The model under review builds one solid part; all positions refer to its coordinate system, in mm. Face numbers are marked on the shaded views. A direction names the side the tool comes from. Give positions to 0.01 mm unless a question says otherwise; leave off trailing zeros. Write each loop counter-clockwise with the first axis right and the second up, starting at its lowest first coordinate (ties: lowest second). Pieces come first, ordered by that corner, then holes. Notation, with made-up numbers: (46, -5) - (72, -5) arc R9 cw to (72, 10) - close; hole circle Ø4 at (-28, 85). An arc over 180 degrees is marked (long way). Write item = value, one per line.
```python
from build123d import *

# Parameters (mm, degrees)
SKETCH002_W  = 48.5
SKETCH002_H  = 45
PAD_DEPTH    = 10
SKETCH003_W  = 42.5
SKETCH003_H  = 24.5
PAD002_DEPTH = 3
SKETCH004_W  = 17.5
SKETCH004_H  = 18
PAD003_DEPTH = 12
FILLET_R     = 1
FILLET001_R  = 8.5


with BuildPart() as part:
    # Sketch002 → Pad (new body)
    with BuildSketch(Plane.XZ):
        Rectangle(SKETCH002_W, SKETCH002_H)
    extrude(amount=PAD_DEPTH)

    # Sketch003 (on Face6 of Pad) → Pad002 (join)
    with BuildSketch(Plane.XZ.offset(10)):
        with Locations((0, 8.25)):
            Rectangle(SKETCH003_W, SKETCH003_H)
    extrude(amount=PAD002_DEPTH)

    # Sketch004 (on Face4 of Pad002) → Pad003 (join)
    with BuildSketch(Plane(origin=(0, 0, 0), x_dir=(1, 0, 0), z_dir=(0, 1, 0))):
        with Locations((0, 12)):
            Rectangle(SKETCH004_W, SKETCH004_H)
    extrude(amount=PAD003_DEPTH)

    # Fillet
    fillet_edges = [part.edges().sort_by_distance(p)[0] for p in [
        (24.25, -5, 22.5),
        (24.25, -5, -22.5),
        (-24.25, -5, 22.5),
        (-24.25, -5, -22.5),
    ]]
    fillet(fillet_edges, radius=FILLET_R)

    # Fillet001
    fillet001_edges = [part.edges().sort_by_distance(p)[0] for p in [
        (8.75, 6, -3),
        (-8.75, 6, -3),
    ]]
    fillet(fillet001_edges, radius=FILLET001_R)


with BuildPart() as part_1:
    # Body placement: moved
    add(part.part.moved(Location((0, 10, 0))))


solid = part_1.part
```
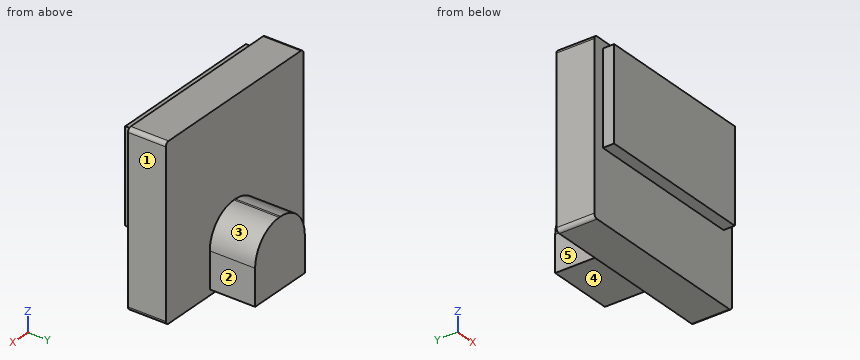
1. Take a section at D-D on x = 7.5. Give the boundary of the cut face in (y, z), and give its area (3 significant figures).
Findings below:
outline = (-3, -4) - (0, -4) - (0, -22.5) - (10, -22.5) - (10, -21) - (22, -21) - (22, -7.06) - (10, -7.06) - (10, 22.5) - (0, 22.5) - (0, 20.5) - (-3, 20.5) - close
area = 691 mm²
2. For line 1 (Y direction, x = -13, z = 11); line 2 (Y direction, x = -15, z = -8.5); line 3 (X direction, y = 15.25, z = -18), list the stretches that pass through material, from the lowest coordinate up. Write a range as from..to.
Findings below:
line_1 = -3..10
line_2 = 0..10
line_3 = -8.75..8.75
3. Take a section at B-B on z = 11.5. Give the boundary of the cut face in (x, y).
Findings below:
outline = (-24.25, 0) - (-21.25, 0) - (-21.25, -3) - (21.25, -3) - (21.25, 0) - (24.25, 0) - (24.25, 10) - (-24.25, 10) - close
4. Take a section at A-A on y = 19. Give the boundary of the cut face in (x, z), and give its area (3 significant figures).
Findings below:
outline = (-8.75, -21) - (8.75, -21) - (8.75, -11.5) arc R8.5 ccw to (0.25, -3) - (-0.25, -3) arc R8.5 ccw to (-8.75, -11.5) - close
area = 284 mm²
5. Machinability: for the marked faces 1, 2, 3, 4 and 5, which of the approach directions +Z, -Z, +X, -X, +Y, -Y give a long, thin tool a straight path to every point of the face, cutting with its end or side? Answer none if there is none.
Findings below:
face_1 = +Z, -Z, +X, +Y, -Y
face_2 = +Z, -Z, +X, +Y
face_3 = +Z, +X, +Y
face_4 = -Z, +X, -X, +Y
face_5 = +Z, -Z, -X, +Y
6. Take a section at C-C on x = -20. Give the boundary of the cut face in (y, z), and give its area (4 significant figures).
Findings below:
outline = (-3, -4) - (0, -4) - (0, -22.5) - (10, -22.5) - (10, 22.5) - (0, 22.5) - (0, 20.5) - (-3, 20.5) - close
area = 523.5 mm²
7. Insertion check: P1, Ø9.5, axis at x = 0.5, y = 17.5, coming from the -Z side; P2, Ø3.5, axis at y = -2, z = 6, coming from the -X side; P3, Ø12, axis at x = -3, z = 5, coming from the +Y side. Each pin has a flat end and moves straight along its axis. Give the tip position at first contact, or say it passes through.
Findings below:
P1 = -21
P2 = -21.25
P3 = 10
